Autodesk Fusion 360 part; units mm, degrees
sketch "Base 1" plane through (0, 0, 0) normal (0, 0, 1) x (1, 0, 0)
  line L0 (6.4814, 44) -> (-33.5, 44)
  line L1 (-33.5, 44) -> (-33.5, -44)
  line L2 (-33.5, -44) -> (6.4814, -44)
  line L3 (-33.5, -25) -> (-33.5, 25) construction
  line L4 (45.8485, -14.44) -> (14.9304, -40.88)
  line L5 (33.5, 25) -> (45.8485, 14.44) construction
  line L6 (14.9304, 40.88) -> (45.8485, 14.44)
  arc A0 (6.4814, -44) -> (14.9304, -40.88) centre (6.4814, -31) ccw
  arc A1 (14.9304, 40.88) -> (6.4814, 44) centre (6.4814, 31) ccw
  circle A2 centre (-2.5, -25) radius 5.3151
  circle A3 centre (-2.5, 25) radius 5.3151
  arc A4 (45.8485, -14.44) -> (45.8485, 14.44) centre (33.5, 0) ccw
  dimension "d2" = 88
  dimension "d4" = 50
  dimension "d6" = 38
  dimension "d7" = 13
  dimension "d8" = 13
  dimension "d9" = 31
  dimension "d10" = 10.6301
extrude "Extrude1" add sketch "Base 1" along normal blind 10
sketch "Base 2" plane through (0, 0, 10) normal (0, 0, 1) x (-1, 0, 0)
  circle A0 centre (2.5, 25) radius 5.3151
  circle A1 centre (2.5, -25) radius 5.3151
  arc A2 (-14.9304, -40.88) -> (-6.4814, -44) centre (-6.4814, -31) ccw
  line L0 (-6.4814, -44) -> (33.5, -44)
  line L1 (33.5, -44) -> (33.5, 44)
  line L2 (33.5, 44) -> (-6.4814, 44)
  arc A3 (-6.4814, 44) -> (-14.9304, 40.88) centre (-6.4814, 31) ccw
  line L3 (-14.9304, 40.88) -> (-45.8485, 14.44)
  arc A4 (-45.8485, 14.44) -> (-45.8485, -14.44) centre (-33.5, 0) ccw
  line L4 (-45.8485, -14.44) -> (-14.9304, -40.88)
  line L5 (33.5, -44) -> (46.5, -44)
  line L6 (46.5, -44) -> (46.5, -25)
  line L7 (46.5, 44) -> (33.5, 44)
  line L8 (33.5, 44) -> (33.5, 19)
  line L9 (30.5, 16) -> (30.5, 16)
  line L10 (30.5, -16) -> (30.5, -16)
  arc A5 (30.5, 16) -> (33.5, 19) centre (30.5, 19) ccw
  line L11 (33.5, -44) -> (33.5, -19)
  arc A6 (33.5, -19) -> (30.5, -16) centre (30.5, -19) ccw
  circle A7 centre (52.5, 0) radius 9.5
  line L12 (52.5, -19) -> (52.5, -19) construction
  arc A8 (52.5, -19) -> (46.5, -25) centre (52.5, -25) ccw
  line L13 (46.5, 25) -> (46.5, 44)
  line L14 (52.5, 19) -> (52.5, 19) construction
  arc A9 (46.5, 25) -> (52.5, 19) centre (52.5, 25) ccw
  line L15 (27, -5) -> (30.5, -5) construction
  line L16 (27, 5) -> (27, -5) construction
  line L17 (30.5, -5) -> (27, -5)
  line L18 (27, -5) -> (27, 5)
  line L19 (27, 5) -> (30.5, 5)
  line L20 (30.5, -16) -> (30.5, -5)
  line L21 (30.5, 5) -> (30.5, 16)
  arc A10 (52.5, -19) -> (52.5, 19) centre (52.5, 0) ccw
  line L22 (26.5, -46.8903) -> (26.5, -44) construction
  line L23 (26.5, 44) -> (26.5, 65) construction
  line L24 (30.5, 5) -> (27, 5) construction
  point P0 (30.5, 0)
  dimension "d13" = 13
  dimension "d14" = 88
  dimension "d17" = 3
  dimension "d18" = 3
  dimension "d20" = 19
  dimension "d21" = 38
  dimension "d22" = 6
  dimension "d23" = 6
extrude "Extrude2" add sketch "Base 2" against normal blind 10 contours L1 L5 L6 L7 L8 L11 A8 L13 A9 A10
extrude "Extrude3" add sketch "Base 2" along normal blind 40 contours L1 L5 L6 L7 L8 L11 A8 L13 A9 A10
extrude "Extrude4" add sketch "Base 2" along normal blind 40 contours L1 A5 A6 L17 L18 L19 L20 L21
sketch "Triangle" plane through (0, 0, 0) normal (0, 1, 0) x (1, 0, 0)
  line L0 (-27, -10) -> (40, -10)
  line L1 (40, -10) -> (-27, -50)
  line L2 (-27, -50) -> (-27, -10)
  dimension "d32" = 67
extrude "Extrude5" add sketch "Triangle" along normal mid plane 10
Build history of the part. All positions in model axes, mm. A direction names the side the tool comes from. Round coordinates to 2 decimals unless told otherwise and drop trailing zeros. Loops run counter-clockwise (first coordinate to the right, second up) from the corner with the lowest first, then second, coordinate; pieces in that order, holes last. Notation, with made-up numbers: (9.5, -31) -> (20.5, -31) arc R11 cw to (20.5, -18) -> close; hole circle Ø11 at (-10.75, 87.5). An arc over 180 degrees is marked (long way). One line per item, written item: value. Start each with the question number.
Q1. Probe line 1 along Y through (x, z) = (-2.5, 5.5); line 2 along Y through (x, z) = (-52.5, 18.5); line 3 along Y through (x, z) = (-10.5, 15). List the from-to ranges inside material, lowest first.
Q2. Cut at C-C on z = 6. List the corners of the cut face in (x, y).
Q3. 3-axis set-ups, long thin cutter, end or side, ignore diameter. For faces 1 (the face through (-46.5, -34, 25)), 2 (the face through (-32.64, -16.9, 29.72)), 3 (the face through (-30.5, 11, 30)): which of +Z, -Z, +X, -X, +Y, -Y reach the whole face in a straight line?
Q4. Two-plate mould, pull along Y, no slides. Class faces 4 (the face through (-4, 5, 25)), 5 (the face through (-61.561, 2.854, 24.65)), 6 (the face through (-32, -44, 8)), 7 (the face through (-46.5, 35, 25)): released by +Y, released by -Y, zero draft, split by the parting line, or undercut.
Q5. Drop flat-ended pins along their axis: pin 1 Ø21 at (y, z) = (36.5, 14.5) entering from -X; pin 2 Ø4 at (x, z) = (-8.5, 23.5) entering from +Y; pin 3 Ø9 at (y, z) = (-11.5, 31) entering from +X. Give the stop position or say it passes through.
Q6. Cut at B-B on z = 42. List the corners of the cut face in (x, y), plus the area to 3 significant figures.
Q7. Cut at D-D on x = -2.5. List the corners of the cut face in (y, z), plus the area to 3 significant figures.
Q8. Cut at A-A on y = 0. List the corners of the cut face in (x, z).
Computed:
1. line 1: -44 to -30.32, -19.68 to 19.68, 30.32 to 44
1. line 2: -19 to -9.5, 9.5 to 19
1. line 3: -5 to 5
2. outline: (-52.5, -19) arc R6 cw to (-46.5, -25) -> (-46.5, -44) -> (6.48, -44) arc R13 ccw to (14.93, -40.88) -> (45.85, -14.44) arc R19 ccw to (45.85, 14.44) -> (14.93, 40.88) arc R13 ccw to (6.48, 44) -> (-46.5, 44) -> (-46.5, 25) arc R6 cw to (-52.5, 19) arc R19 ccw to start; hole circle Ø19 at (-52.5, 0); hole circle Ø10.63 at (-2.5, -25); hole circle Ø10.63 at (-2.5, 25)
3. face 1: +Z, -Z, -X, -Y
3. face 2: +Z, +X, -Y
3. face 3: +Z, +X, +Y
4. face 4: released by +Y
4. face 5: undercut
4. face 6: released by -Y
4. face 7: zero draft
5. pin 1: x = -46.5
5. pin 2: y = 5
5. pin 3: x = -30.5
6. outline: (-52.5, -19) arc R6 cw to (-46.5, -25) -> (-46.5, -44) -> (-33.5, -44) -> (-33.5, -19) arc R3 cw to (-30.5, -16) -> (-30.5, -5) -> (-13.6, -5) -> (-13.6, 5) -> (-30.5, 5) -> (-30.5, 16) arc R3 cw to (-33.5, 19) -> (-33.5, 44) -> (-46.5, 44) -> (-46.5, 25) arc R6 cw to (-52.5, 19) arc R19 ccw to start; hole circle Ø19 at (-52.5, 0)
6. area: 1,940 mm²
7. outline: (-44, 0) -> (-30.32, 0) -> (-30.32, 10) -> (-44, 10) -> close; (-19.68, 0) -> (19.68, 0) -> (19.68, 10) -> (5, 10) -> (5, 35.37) -> (-5, 35.37) -> (-5, 10) -> (-19.68, 10) -> close; (30.32, 0) -> (44, 0) -> (44, 10) -> (30.32, 10) -> close
7. area: 921 mm²
8. outline: (-71.5, 0) -> (-62, 0) -> (-62, 50) -> (-71.5, 50) -> close; (-43, 0) -> (52.5, 0) -> (52.5, 10) -> (40, 10) -> (-27, 50) -> (-43, 50) -> close
